Could you check a few things on this model? Use its own coordinates, in mm. Face numbers are marked on the shaded views. A direction names the side the tool comes from. Give positions to 0.01 mm unless a question says otherwise; leave off trailing zeros. Loops run counter-clockwise (first coordinate to the right, second up) from the corner with the lowest first, then second, coordinate; pieces in that order, holes last. Notation, with made-up numbers: (52.5, 37) - (96.5, 37) arc R11 ccw to (96.5, 56) - close; hole circle Ø11 at (-9, 9.5). An arc over 180 degrees is marked (long way). Answer in a Markdown table with one row per item. Add a question column.
```python
from build123d import *

# Parameters (mm, degrees)
SKETCH2_R          = 0.725
CUT_EXTRUDE1_DEPTH = 18.567344705


with BuildPart() as part:
    # Sketch1 → Revolve1 (revolve)
    with BuildSketch(Plane.XY, mode=Mode.PRIVATE) as revolve1_sk:
        Polygon((-3.75, 0), (-12, 0), (-12, -2), (-4.44, -2), (-4.44, -4.54), (-2.65, -4.54), (-2.65, -1.54), (-1.4, -1.54), (-1.4, -0.8), (-3, -0.8), (-3, 0.4), (-3.75, 0.4), align=None)
    revolve(revolve1_sk.sketch.rotate(Axis((0, 0, 0), (0, -1, 0)), 270), axis=Axis((0, 0, 0), (0, -1, 0)))

    # Sketch2 → Cut-Extrude1 (cut, through all)
    with BuildSketch(Plane(origin=(0, 0, 0), x_dir=(1, 0, 0), z_dir=(0, 1, 0))):
        with Locations(Location((-8.25, 0, 0), (0, 0, 270))):
            Circle(SKETCH2_R)
        with Locations(Location((-7.752464121, 2.821666182, 0), (0, 0, 270))):
            Circle(SKETCH2_R)
        with Locations(Location((0, 7, 0), (0, 0, 270))):
            Circle(SKETCH2_R)
        with Locations(Location((0, 9.9, 0), (0, 0, 270))):
            Circle(SKETCH2_R)
        with Locations(Location((2.394141003, 6.577848346, 0), (0, 0, 270))):
            Circle(SKETCH2_R)
        with Locations(Location((3.385999419, 9.302956946, 0), (0, 0, 270))):
            Circle(SKETCH2_R)
        with Locations(Location((-2.394141003, 6.577848346, 0), (0, 0, 90))):
            Circle(SKETCH2_R)
        with Locations(Location((-3.385999419, 9.302956946, 0), (0, 0, 90))):
            Circle(SKETCH2_R)
        with Locations(Location((-7.752464121, -2.821666182, 0), (0, 0, 90))):
            Circle(SKETCH2_R)
        with Locations(Location((7.752464121, -2.821666182, 0), (0, 0, 270))):
            Circle(SKETCH2_R)
        with Locations(Location((7.752464121, 2.821666182, 0), (0, 0, 90))):
            Circle(SKETCH2_R)
        with Locations(Location((8.25, 0, 0), (0, 0, 270))):
            Circle(SKETCH2_R)
        with Locations(Location((2.394141003, -6.577848346, 0), (0, 0, 90))):
            Circle(SKETCH2_R)
        with Locations(Location((3.385999419, -9.302956946, 0), (0, 0, 90))):
            Circle(SKETCH2_R)
        with Locations(Location((0, -9.9, 0), (0, 0, 270))):
            Circle(SKETCH2_R)
        with Locations(Location((0, -7, 0), (0, 0, 270))):
            Circle(SKETCH2_R)
        with Locations(Location((-2.394141003, -6.577848346, 0), (0, 0, 270))):
            Circle(SKETCH2_R)
        with Locations(Location((-3.385999419, -9.302956946, 0), (0, 0, 270))):
            Circle(SKETCH2_R)
    extrude(amount=-CUT_EXTRUDE1_DEPTH, mode=Mode.SUBTRACT)


solid = part.part
```
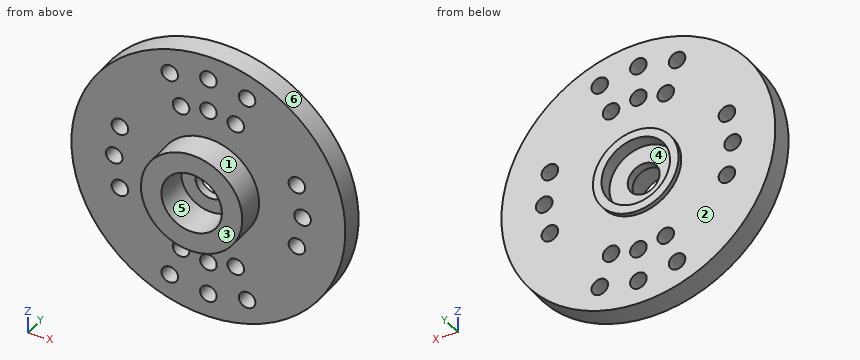
(1) On a 3-axis mill with a long thin cutter (end or side, diameter ignored), from which of +Z, -Z, +X, -X, +Y, -Y can I reach the whole of each face in a straight line? I mean the marked faces 1 and 2. Say none if no direction works.
(2) We'd pull the mould along X, two halves only. Please class the marked faces 3, 4, 5 and 6: pulls with the +X half, pulls with the -X half, needs draft (parallel to the pull), parting line crosses it, or undercut.
(3) For pin 1 Ø1.9 at (x, z) = (-3.39, 9.3) entering from +Y; pin 2 Ø1.9 at (x, z) = (8.25, 0) entering from -Y, each with a flat end and sliding along its axis, tell me the tip position at first contact or that it passes through.
(4) Please list where these lines run through material, in increasing order: line 1 (X direction, y = -0.45, z = 0) (3 decimals); line 2 (Y direction, x = -0.5, z = -8.25); line 3 (Z direction, x = 1.5, y = -3.05).
(5) I want a section at A-A on z = 0. State how many separate pieces and enclosed holes the cut face has, then the cut area to 3 significant figures.
(6) I want a section at D-D on x = -4.75. Please give me the cut outline in (y, z), then the cut area to 3 significant figures.
(7) I want a section at B-B on y = -2.3. Please give me the cut outline in (x, z).
(8) I want a section at C-C on z = -7. Please give me the cut outline in (x, y) (3 decimals).
Reported:
| question | item | result |
|---|---|---|
| 1 | face 1 | -Y |
| 1 | face 2 | +Y |
| 2 | face 3 | needs draft |
| 2 | face 4 | undercut |
| 2 | face 5 | undercut |
| 2 | face 6 | parting line crosses it |
| 3 | pin 1 | y = 0 |
| 3 | pin 2 | y = -2 |
| 4 | line 1 | -12 to -8.975, -7.525 to -3, 3 to 7.525, 8.975 to 12 |
| 4 | line 2 | -2 to 0 |
| 4 | line 3 | -4.18 to -2.18, 2.18 to 4.18 |
| 5 | separate pieces | 4 |
| 5 | enclosed holes | 0 |
| 5 | area | 42.6 mm² |
| 6 | outline | (-2, -11.02) - (0, -11.02) - (0, 11.02) - (-2, 11.02) - close |
| 6 | area | 44.1 mm² |
| 7 | outline | circle Ø8.88 at (0, 0); hole circle Ø5.3 at (0, 0) |
| 8 | outline | (-9.747, -2) - (-2.984, -2) - (-2.984, 0) - (-9.747, 0) - close; (-1.805, -2) - (-0.725, -2) - (-0.725, 0) - (-1.805, 0) - close; (0.725, -2) - (1.805, -2) - (1.805, 0) - (0.725, 0) - close; (2.984, -2) - (9.747, -2) - (9.747, 0) - (2.984, 0) - close |
